Input: part model. Units: mm. Frame: model coordinates. A direction names the side the tool comes from. Give positions to 0.01 mm unless a question says otherwise; leave off trailing zeros. Loops run counter-clockwise (first coordinate to the right, second up) from the corner with the lowest first, then second, coordinate; pieces in that order, holes last. Notation, with made-up numbers: M -2,52 L 5,52 A30 ccw 5,85 Z; hole C 11.5,15 d11. An arc over 180 degrees is marked long. One line per item, written item: value. Start each with the question number.
(1) Access query for faces 5 (the flat face through (0, 1, 10.25)), 6 (the flat face through (-15, 5, 5.75)), 7 (the flat face through (0, 1, -10.25)), 8 (the flat face through (14.3, 2, 0)). Directions: +Z, -Z, +X, -X, +Y, -Y. A direction counts if a zero-diameter tool reaches every point of the face in a straight line with its end or side. Return the directions, or none.
(2) Ray query, line 1 along Z through (x, y) = (-14.7, 4.8); line 2 along Z through (x, y) = (-0.5, 1.75); line 3 along X through (y, z) = (4.5, -15.25). Return the intervals inside material, ascending. Write a range as from..to.
(3) Pin query (flat end, axial travel): P1, Ø0.9, axis at x = 5.5, y = 1, coming from the +Z side; P2, Ø3, axis at x = -15, z = -16, coming from the -Y side; P3, Ø1, axis at x = 0.5, z = -10.5, coming from the +Y side. Return the tip coordinate at first contact, or that it passes through.
(4) Section C-C on z = -15.25. Output: boundary loops of the cut face in (x, y).
(5) Section D-D on x = 1.5. Output: boundary loops of the cut face in (y, z), plus the area to 3 significant figures.
(6) Section A-A on y = 5.75. Output: boundary loops of the cut face in (x, z).
(7) Section B-B on x = -14.7. Output: boundary loops of the cut face in (y, z), plus the area to 3 significant figures.
(8) Pull-direction query (X, two-part tool) for faces 1 (the flat face through (-9.7, 5, -13)), 2 (the flat face through (-2, 2, 5.3)), 3 (the flat face through (-15, 5, -20.25)), 4 (the cylindrical face through (-14.146, 5.268, 16.315)); classes: released by +X, released by -X, zero draft, split by the parting line, or undercut.
```python
from build123d import *

# Parameters (mm, degrees)
SKETCH1_W                                       = 39.4
SKETCH1_H                                       = 20.5
BOSS_EXTRUDE1_DEPTH                             = 3
SKETCH3_W                                       = 28.6
SKETCH3_H                                       = 10.6
CUT_EXTRUDE1_DEPTH                              = 3
SKETCH4_W                                       = 10
SKETCH4_H                                       = 4.5
BOSS_EXTRUDE2_DEPTH                             = 3.5
SKETCH5_W                                       = 10
SKETCH5_H                                       = 3.5
BOSS_EXTRUDE3_DEPTH                             = 10
SKETCH6_W                                       = 10
SKETCH6_H                                       = 3.5
BOSS_EXTRUDE4_DEPTH                             = 10
CSK_FOR_M2_FLAT_HEAD_MACHINE_SCREW1_D           = 2.4
CSK_FOR_M2_FLAT_HEAD_MACHINE_SCREW1_CSINK_D     = 4.4
CSK_FOR_M2_FLAT_HEAD_MACHINE_SCREW1_CSINK_ANGLE = 90
CSK_FOR_M2_FLAT_HEAD_MACHINE_SCREW2_D           = 2.4
CSK_FOR_M2_FLAT_HEAD_MACHINE_SCREW2_CSINK_D     = 4.4
CSK_FOR_M2_FLAT_HEAD_MACHINE_SCREW2_CSINK_ANGLE = 90
SKETCH16_W                                      = 2.9
SKETCH16_H                                      = 10.6
CUT_EXTRUDE2_DEPTH                              = 3


with BuildPart() as part:
    # Sketch1 → Boss-Extrude1 (new body)
    with BuildSketch(Plane(origin=(0, 0, 0), x_dir=(1, 0, 0), z_dir=(0, 1, 0))):
        Rectangle(SKETCH1_W, SKETCH1_H)
    extrude(amount=BOSS_EXTRUDE1_DEPTH)

    # Sketch3 → Cut-Extrude1 (cut)
    with BuildSketch(Plane(origin=(0, 3, 0), x_dir=(1, 0, 0), z_dir=(0, 1, 0))):
        Rectangle(SKETCH3_W, SKETCH3_H)
    extrude(amount=-CUT_EXTRUDE1_DEPTH, mode=Mode.SUBTRACT)

    # Sketch4 → Boss-Extrude2 (add)
    with BuildSketch(Plane(origin=(0, 3, 0), x_dir=(1, 0, 0), z_dir=(0, 1, 0))):
        with Locations((-14.7, 8)):
            Rectangle(SKETCH4_W, SKETCH4_H)
        with Locations((-14.7, -8)):
            Rectangle(SKETCH4_W, SKETCH4_H)
    extrude(amount=BOSS_EXTRUDE2_DEPTH)

    # Sketch5 → Boss-Extrude3 (add)
    with BuildSketch(Plane.XY.offset(10.25)):
        with Locations((-14.7, 4.75)):
            Rectangle(SKETCH5_W, SKETCH5_H)
    extrude(amount=BOSS_EXTRUDE3_DEPTH)

    # Sketch6 → Boss-Extrude4 (add)
    with BuildSketch(Plane(origin=(0, 0, -10.25), x_dir=(-1, 0, 0), z_dir=(0, 0, -1))):
        with Locations((14.7, 4.75)):
            Rectangle(SKETCH6_W, SKETCH6_H)
    extrude(amount=BOSS_EXTRUDE4_DEPTH)

    # CSK for M2 Flat Head Machine Screw1 (through all)
    with Locations(Plane(origin=(0, 3, 0), x_dir=(-1, 0, 0), z_dir=(0, -1, 0))):
        with Locations((14.7, 15.25)):
            CounterSinkHole(CSK_FOR_M2_FLAT_HEAD_MACHINE_SCREW1_D / 2, CSK_FOR_M2_FLAT_HEAD_MACHINE_SCREW1_CSINK_D / 2, counter_sink_angle=CSK_FOR_M2_FLAT_HEAD_MACHINE_SCREW1_CSINK_ANGLE)

    # CSK for M2 Flat Head Machine Screw2 (through all)
    with Locations(Plane(origin=(0, 3, 0), x_dir=(-1, 0, 0), z_dir=(0, -1, 0))):
        with Locations((14.7, -15.25)):
            CounterSinkHole(CSK_FOR_M2_FLAT_HEAD_MACHINE_SCREW2_D / 2, CSK_FOR_M2_FLAT_HEAD_MACHINE_SCREW2_CSINK_D / 2, counter_sink_angle=CSK_FOR_M2_FLAT_HEAD_MACHINE_SCREW2_CSINK_ANGLE)

    # Sketch16 → Cut-Extrude2 (cut)
    with BuildSketch(Plane(origin=(0, 3, 0), x_dir=(1, 0, 0), z_dir=(0, 1, 0))):
        with Locations((-15.75, 0)):
            Rectangle(SKETCH16_W, SKETCH16_H)
    extrude(amount=-CUT_EXTRUDE2_DEPTH, mode=Mode.SUBTRACT)


solid = part.part
```
Output values:
1. face 5: +Z, +X, -X, -Y
1. face 6: +X, -X, +Y
1. face 7: -Z, +X, -X, -Y
1. face 8: +Y, -Y
2. line 1: z = -20.25..-16.45, -14.05..-5.75, 5.75..14.05, 16.45..20.25
2. line 2: z = -10.25..-5.3, 5.3..10.25
2. line 3: x = -19.7..-15.9, -13.5..-9.7
3. P1: stops at z = 10.25
3. P2: stops at y = 3
3. P3: stops at y = 3
4. outline: M -19.7,3 L -16.9,3 L -15.9,4 L -15.9,6.5 L -19.7,6.5 Z; M -13.5,4 L -12.5,3 L -9.7,3 L -9.7,6.5 L -13.5,6.5 Z
5. outline: M 0,-10.25 L 3,-10.25 L 3,-5.3 L 0,-5.3 Z; M 0,5.3 L 3,5.3 L 3,10.25 L 0,10.25 Z
5. area: 29.7 mm²
6. outline: M -19.7,-20.25 L -9.7,-20.25 L -9.7,-5.75 L -19.7,-5.75 Z; M -19.7,5.75 L -9.7,5.75 L -9.7,20.25 L -19.7,20.25 Z; hole C -14.7,-15.25 d2.4; hole C -14.7,15.25 d2.4
7. outline: M 0,-10.25 L 3,-10.25 L 3,-13.05 L 4,-14.05 L 6.5,-14.05 L 6.5,-5.75 L 3,-5.75 L 3,-5.3 L 0,-5.3 Z; M 0,5.3 L 3,5.3 L 3,5.75 L 6.5,5.75 L 6.5,14.05 L 4,14.05 L 3,13.05 L 3,10.25 L 0,10.25 Z; M 3,-20.25 L 6.5,-20.25 L 6.5,-16.45 L 4,-16.45 L 3,-17.45 Z; M 3,17.45 L 4,16.45 L 6.5,16.45 L 6.5,20.25 L 3,20.25 Z
7. area: 112 mm²
8. face 1: released by +X
8. face 2: undercut
8. face 3: zero draft
8. face 4: undercut
